Source: three-view drawing plus pictorial views. Frame: mm from the lowest corner of the part. A direction names the side the tool comes from. Give positions to 0.01 mm unless a question says otherwise; leave off trailing zeros. Order: outer loops, then holes, each group sorted by start corner. A loop starts at its lowest first (then second) coordinate and runs counter-clockwise, first axis right, second up. Notation, with made-up numbers: (21, 44) -> (42, 44) arc R14 ccw to (42, 57) -> close; hole circle Ø6 at (-22, 12.25). An arc over 180 degrees is marked (long way). Answer in a Markdown table with one row per item. Add a question column.
Q1. Contact query for flat-ended pins moving along their axis: P1, Ø1, axis at x = 9.5, y = 50.5, coming from the -Z side; P2, Ø4, axis at x = 12.5, y = 151, coming from the +Z side (1 decimal); P3, Ø1, axis at x = 8.5, y = 77, coming from the -Z side; P4, Ø8, axis at x = 7.5, z = 12, coming from the -Y side. Output: stop coordinate, or through.
Q2. Cut plane A-A on x = 10. Return the cut outline in (y, z), and give its area (3 significant figures).
Q3. Set-up query: the marked faces 1 and 2. Return all of +Z, -Z, +X, -X, +Y, -Y with unobstructed straight access to the full face (end or side cutting, diameter ignored); none if empty.
Q4. Line query: line 1 along Y through (x, z) = (14.5, 14.25); line 2 along Z through (x, y) = (5.5, 70.5) (1 decimal); line 3 along Z through (x, y) = (8.75, 91). Output: solid intervals per line, ascending. Write a range as from..to.
Q5. Cut plane B-B on y = 60. Return the cut outline in (x, z).
Q6. Cut plane C-C on x = 17. Return the cut outline in (y, z), and give its area (3 significant figures).
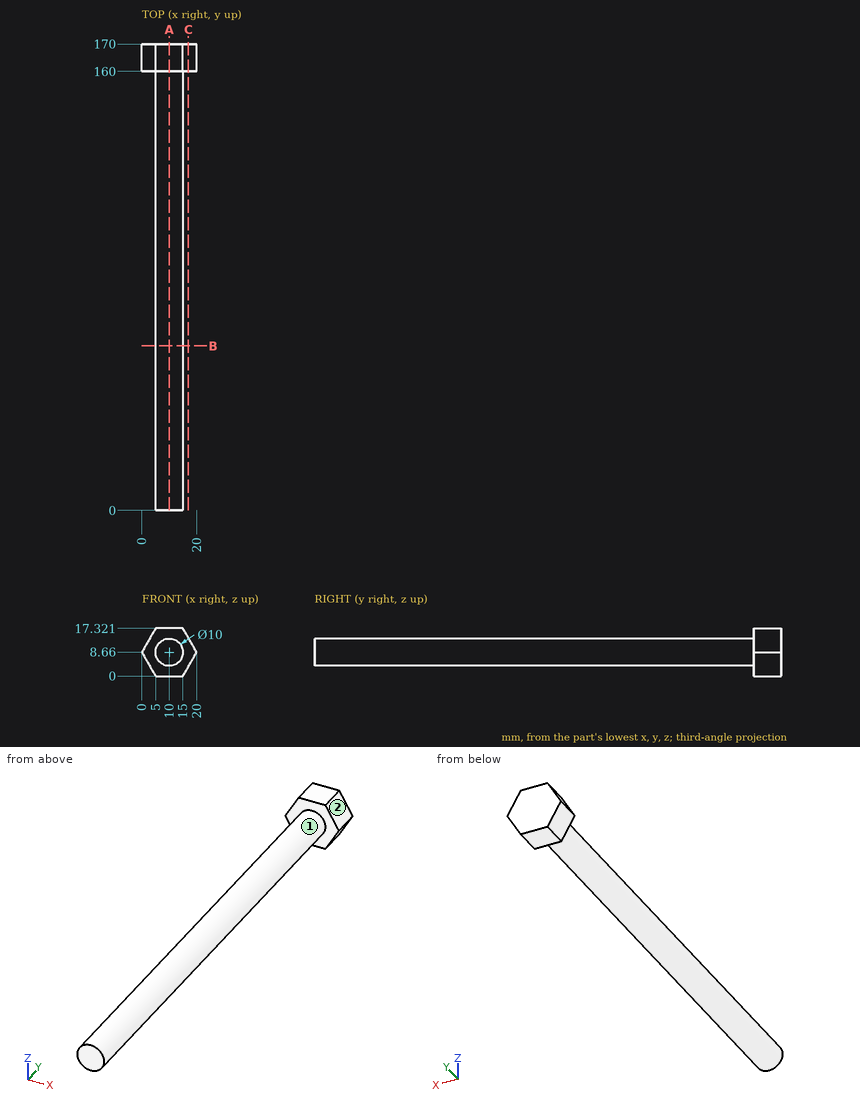
Completed:
| question | item | result |
|---|---|---|
| 1 | P1 | stops at z = 3.66 |
| 1 | P2 | stops at z = 13.6 |
| 1 | P3 | stops at z = 3.76 |
| 1 | P4 | stops at y = 0 |
| 2 | outline | (0, 3.66) -> (160, 3.66) -> (160, 0) -> (170, 0) -> (170, 17.32) -> (160, 17.32) -> (160, 13.66) -> (0, 13.66) -> close |
| 2 | area | 1,770 mm² |
| 3 | face 1 | -Y |
| 3 | face 2 | +Z, +X, +Y, -Y |
| 4 | line 1 | y = 160..170 |
| 4 | line 2 | z = 6.5..10.8 |
| 4 | line 3 | z = 3.82..13.5 |
| 5 | outline | circle Ø10 at (10, 8.66) |
| 6 | outline | (160, 3.46) -> (170, 3.46) -> (170, 13.86) -> (160, 13.86) -> close |
| 6 | area | 104 mm² |
